from build123d import *

# Parameters (mm, degrees)
SKETCH24_R          = 5.4
BOSS_EXTRUDE1_DEPTH = 30
SKETCH26_R          = 4.2
RODS_SLOT_DEPTH     = 62.731822261
SKETCH25_R          = 5.4
RODS_HOLE_DEPTH     = 50


with BuildPart() as part:
    # Sketch24 → Boss-Extrude1 (new body)
    with BuildSketch(Plane(origin=(0, 0, 0), x_dir=(0, 0, -1), z_dir=(1, 0, 0))):
        Polygon((10, -9.157855987), (10, 44.842144013), (-20, 44.842144013), (-20, -29.157855987), (-10, -29.157855987), (-10, -9.157855987), (-2.9, -9.157855987), (-2.9, -12.157855987), (2.9, -12.157855987), (2.9, -9.157855987), align=None)
        with Locations((0, 24.842144013)):
            Circle(SKETCH24_R, mode=Mode.SUBTRACT)
        with Locations((0, 2.842144013)):
            Circle(SKETCH24_R, mode=Mode.SUBTRACT)
    extrude(amount=BOSS_EXTRUDE1_DEPTH)

    # Sketch26 → rods_slot (cut, through all)
    with BuildSketch(Plane.XY.offset(-10)):
        with Locations((15, 44.842144013)):
            Circle(SKETCH26_R)
    extrude(amount=RODS_SLOT_DEPTH, mode=Mode.SUBTRACT)

    # Sketch25 → rods-hole (cut)
    with BuildSketch(Plane.XY.offset(20)):
        with Locations((15, 13.842144013)):
            Circle(SKETCH25_R)
    extrude(amount=-RODS_HOLE_DEPTH, mode=Mode.SUBTRACT)


solid = part.part
Input: part model. Units: mm. Frame: model coordinates. A direction names the side the tool comes from. Give positions to 0.01 mm unless a question says otherwise; leave off trailing zeros. Write each loop counter-clockwise with the first axis right and the second up, starting at its lowest first coordinate (ties: lowest second). Pieces come first, ordered by that corner, then holes. Notation, with made-up numbers: (-17, 46) -> (42, 46) arc R26 ccw to (42, 72) -> close; hole circle Ø8 at (-1, 72). An arc over 180 degrees is marked (long way). Use one line per item in the form item = value. Start each with the question number.
1) Draft query along Z for faces 4 (the flat face through (15, -11, -2.9)), 5 (the flat face through (15, -9.158, -6)), 6 (the flat face through (15, -9.158, 6)). Return one class per face: pulls with the +Z half, pulls with the -Z half, needs draft (parallel to the pull), parting line crosses it, or undercut.
2) Set-up query: faces 1 (the flat face through (15, -11, 2.9)), 2 (the cylindrical face through (14.79, -2.43, 1.17)), 3 (the flat face through (15, -12.158, 0)). Return all of +Z, -Z, +X, -X, +Y, -Y with unobstructed straight access to the full face (end or side cutting, diameter ignored); none if empty.
3) Section query C-C on z = -2. Return the cut outline in (x, y).
4) Ray query, probe 1 along Y at (x, z) = (22.5, 0); probe 2 along Y at (x, z) = (15, 9.75); probe 3 along Y at (x, z) = (15, -1.75). Return the intervals inside material, ascending. Write a range as from..to.
5) Section query A-A on y = -10.5. Return the cut outline in (x, z).
6) Pin query (flat end, axial travel): pin 1 (0.9 mm diameter, centred on x = 9, y = -10.5, fed in from -Z); pin 2 (10 mm diameter, centred on y = 19, z = 13, fed in from -X); pin 3 (1.7 mm diameter, centred on x = 12.5, z = 0.5, fed in from -Y); pin 4 (2 mm diameter, centred on x = 14.5, z = 12.5, fed in from +Y). Return the tip coordinate at first contact, or that it passes through.
7) Section query B-B on x = 15. Return the cut outline in (y, z), then the cut area to 3 significant figures.
8) Section query D-D on z = 13.5. Return the cut outline in (x, y), then the cut area to 3 significant figures.
Outcome:
q1.face_4 = pulls with the -Z half
q1.face_5 = needs draft
q1.face_6 = undercut
q2.face_1 = +X, -X, -Y
q2.face_2 = +X, -X
q2.face_3 = -Z, +X, -X, -Y
q3.outline = (0, -12.16) -> (30, -12.16) -> (30, -2.17) -> (0, -2.17) -> close; (0, 7.86) -> (30, 7.86) -> (30, 19.83) -> (0, 19.83) -> close; (0, 29.86) -> (30, 29.86) -> (30, 44.84) -> (19.2, 44.84) arc R4.2 cw to (10.8, 44.84) -> (0, 44.84) -> close; hole circle Ø10.8 at (15, 13.84)
q4.probe_1 = -12.16..-2.56, 8.24..19.44, 30.24..44.84
q4.probe_2 = -9.16..8.44, 19.24..40.64
q4.probe_3 = -12.16..-2.27, 7.95..8.44, 19.24..19.73, 29.95..40.64
q5.outline = (0, -2.9) -> (30, -2.9) -> (30, 2.9) -> (0, 2.9) -> close; (0, 10) -> (30, 10) -> (30, 20) -> (0, 20) -> close
q6.pin_1 = -2.9
q6.pin_2 = 0
q6.pin_3 = -12.16
q6.pin_4 = 40.92
q7.outline = (-29.16, 10) -> (-9.16, 10) -> (-9.16, 2.9) -> (-12.16, 2.9) -> (-12.16, -2.9) -> (-9.16, -2.9) -> (-9.16, -10) -> (8.44, -10) -> (8.44, 20) -> (-29.16, 20) -> close; (19.24, -10) -> (40.64, -10) -> (40.64, 20) -> (19.24, 20) -> close; hole circle Ø10.8 at (2.84, 0); hole circle Ø10.8 at (24.84, 0)
q7.area = 1,200 mm^2
q8.outline = (0, -29.16) -> (30, -29.16) -> (30, 44.84) -> (19.2, 44.84) arc R4.2 cw to (10.8, 44.84) -> (0, 44.84) -> close; hole circle Ø10.8 at (15, 13.84)
q8.area = 2,100 mm^2
